Work out the finished part from the listing and answer in its coordinate system (mm). Round coordinates to 2 decimals unless told otherwise and drop trailing zeros. Write each loop counter-clockwise with the first axis right and the second up, starting at its lowest first coordinate (ties: lowest second). Pieces come first, ordered by that corner, then holes. Notation, with made-up numbers: (44, 26.5) -> (101, 26.5) arc R5 cw to (101, 33.5) -> close; hole circle Ø11 at (43.25, -35). An arc over 180 degrees is marked (long way). Answer as a JSON object with one key per item and string values. Group by question number.
from build123d import *

# Parameters (mm, degrees)
EXTRUDE_1_DEPTH      = 3
CUT_EXTRUDE_2_DEPTH  = 10
SKETCH_4_R           = 1.5
CUT_EXTRUDE_3_DEPTH  = 10
CUT_EXTRUDE_6_DEPTH  = 327.235911434
SKETCH_12_W          = 293.771267283
SKETCH_12_H          = 20
EXTRUDE_2_DEPTH      = 3
SKETCH_13_R          = 2
CUT_EXTRUDE_9_DEPTH  = 278.623703749
CUT_EXTRUDE_10_DEPTH = 10
MM_2_D               = 1.5
CUT_EXTRUDE_11_DEPTH = 278.623703749
MM_3_D               = 1.5
FILLET_1_R           = 2


with BuildPart() as part:
    # 草图1 → 凸台-拉伸1 (new body)
    with BuildSketch(Plane.XY):
        Polygon((-31.770103996, 71.767703031), (318.229896004, 71.767703031), (292.931935015, -47.249845949), (-31.770103996, 21.767703031), align=None)
    extrude(amount=EXTRUDE_1_DEPTH)

    # 草图3 → 切除-拉伸2 (cut)
    with BuildSketch(Plane.XY.offset(3)):
        Polygon((-0.469380772, 15.114528924), (0.1543543, 18.048971727), (-31.770103996, 24.834724815), (-31.770103996, 21.767703031), align=None)
        Polygon((176.220922432, -19.375132621), (205.565350454, -25.612483345), (204.941615382, -28.546926147), (175.59718736, -22.309575423), align=None)
    extrude(amount=-CUT_EXTRUDE_2_DEPTH, mode=Mode.SUBTRACT)

    # 草图4 → 切除-拉伸3 (cut)
    with BuildSketch(Plane.XY.offset(3)):
        with Locations((-20.141101902, 42.809716012)):
            Circle(SKETCH_4_R)
        with Locations((-0.578149887, 38.651482195)):
            Circle(SKETCH_4_R)
        with Locations((185.269894252, -0.85173906)):
            Circle(SKETCH_4_R)
        with Locations((204.832846267, -5.009972876)):
            Circle(SKETCH_4_R)
    extrude(amount=-CUT_EXTRUDE_3_DEPTH, mode=Mode.SUBTRACT)

    # 草图7 → 切除-拉伸6 (cut, through all)
    with BuildSketch(Plane.XY.offset(3)):
        Polygon((292.931935015, -47.249845949), (239.133816975, -35.814702954), (262.001163287, 71.767703031), (318.229896004, 71.767703031), align=None)
    extrude(amount=-CUT_EXTRUDE_6_DEPTH, mode=Mode.SUBTRACT)

    # 草图12 → 凸台-拉伸2 (add)
    with BuildSketch(Plane.XY.offset(3)):
        with Locations((115.115529646, 81.767703031)):
            Rectangle(SKETCH_12_W, SKETCH_12_H)
    extrude(amount=-EXTRUDE_2_DEPTH)

    # 草图13 → 切除-拉伸9 (cut, through all)
    with BuildSketch(Plane.XY.offset(3)):
        with Locations((-6.770103996, 81.767703031)):
            Circle(SKETCH_13_R)
        with Locations((73.229896004, 81.767703031)):
            Circle(SKETCH_13_R)
        with Locations((153.229896004, 81.767703031)):
            Circle(SKETCH_13_R)
        with Locations((233.229896004, 81.767703031)):
            Circle(SKETCH_13_R)
    extrude(amount=-CUT_EXTRUDE_9_DEPTH, mode=Mode.SUBTRACT)

    # 草图14 → 切除-拉伸10 (cut)
    with BuildSketch(Plane.XY.offset(3)):
        with BuildLine():
            Line((33.229896004, 67.767703031), (213.229896004, 67.767703031))
            ThreePointArc((213.229896004, 67.767703031), (221.229896004, 59.767703031), (213.229896004, 51.767703031))
            Line((213.229896004, 51.767703031), (33.229896004, 51.767703031))
            ThreePointArc((33.229896004, 51.767703031), (25.229896004, 59.767703031), (33.229896004, 67.767703031))
        make_face()
        with BuildLine():
            Line((53.229896004, 35.767703031), (223.229896004, 35.767703031))
            ThreePointArc((223.229896004, 35.767703031), (229.229896004, 29.767703031), (223.229896004, 23.767703031))
            Line((223.229896004, 23.767703031), (53.229896004, 23.767703031))
            ThreePointArc((53.229896004, 23.767703031), (47.229896004, 29.767703031), (53.229896004, 35.767703031))
        make_face()
    extrude(amount=-CUT_EXTRUDE_10_DEPTH, mode=Mode.SUBTRACT)

    # 大小mm 暗销槽口2 (through all)
    with Locations(Plane.XY.offset(3)):
        with Locations((0.1543543, 18.048971727), (176.220922432, -19.375132621), (205.565350454, -25.612483345)):
            Hole(MM_2_D / 2)

    # 草图18 → 切除-拉伸11 (cut, through all)
    with BuildSketch(Plane(origin=(0, 0, 0), x_dir=(-1, 0, 0), z_dir=(0, 0, -1))):
        Polygon((-152.291642964, -11.221785469), (-151.667907892, -14.156228271), (-122.32347987, -7.918877547), (-122.947214942, -4.984434744), align=None)
        Polygon((-64.258358898, 7.490266705), (-63.634623826, 4.555823902), (-34.290195804, 10.793174627), (-34.913930876, 13.727617429), align=None)
    extrude(amount=-CUT_EXTRUDE_11_DEPTH, mode=Mode.SUBTRACT)

    # 大小mm 暗销槽口3 (through all)
    with Locations(Plane(origin=(0, 0, 0), x_dir=(-1, 0, 0), z_dir=(0, 0, -1))):
        with Locations((-152.291642964, -11.221785469), (-151.667907892, -14.156228271), (-122.32347987, -7.918877547), (-122.947214942, -4.984434744), (-64.258358898, 7.490266705), (-63.634623826, 4.555823902), (-34.290195804, 10.793174627), (-34.913930876, 13.727617429)):
            Hole(MM_3_D / 2)

    # 圆角1
    fillet_1_edges = [part.edges().sort_by_distance(p)[0] for p in [
        (-31.770103996, 24.834724815, 1.5),
        (239.133816975, -35.814702954, 1.5),
        (262.001163287, 71.767703031, 1.5),
        (-31.770103996, 91.767703031, 1.5),
        (262.001163287, 91.767703031, 1.5),
    ]]
    fillet(fillet_1_edges, radius=FILLET_1_R)


solid = part.part
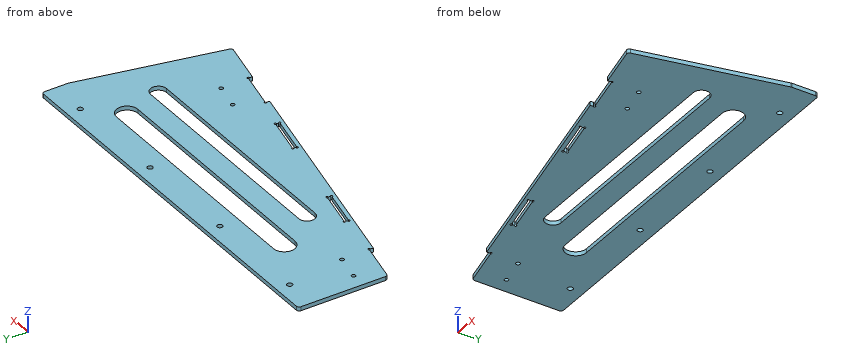
1) A cutting plane is placed at D-D on z = 2.1. State how many separate pieces and enclosed holes the cut face has, plus the area to 3 significant figures.
2) A cutting plane is placed at B-B on x = 168.5. Determine the outline of the cut face in (y, z), plus the area to 3 significant figures.
3) A cutting plane is placed at C-C on x = 137. Determine the outline of the cut face in (y, z), plus the area to 3 significant figures.
4) Straight lines are drawn through the part: L1, parallel to Y at x = 179.5, z = 0.5; L2, parallel to Y at x = 93, z = 0.9; L3, parallel to Y at x = 139, z = 1.1. For each, find the intervals that lie inside material, in ascending order.
5) A cutting plane is placed at A-A on y = 56. Determine the outline of the cut face in (x, z).
6) This flat-tipped pin is pushed along its axis until it touches: P1, Ø1, axis at y = 63.5, z = 0.5, coming from the +X side. Where does it stop, or does it pass through?
Established:
{
 "1": {"separate pieces": "1", "enclosed holes": "12", "area": "22,800 mm²"},
 "2": {"outline": "(-20.8, 0) -> (23.77, 0) -> (23.77, 3) -> (-20.8, 3) -> close; (35.77, 0) -> (51.77, 0) -> (51.77, 3) -> (35.77, 3) -> close; (67.77, 0) -> (91.77, 0) -> (91.77, 3) -> (67.77, 3) -> close", "area": "254 mm²"},
 "3": {"outline": "(-14.11, 0) -> (-11.04, 0) -> (-11.04, 3) -> (-14.11, 3) -> close; (-7.97, 0) -> (23.77, 0) -> (23.77, 3) -> (-7.97, 3) -> close; (35.77, 0) -> (51.77, 0) -> (51.77, 3) -> (35.77, 3) -> close; (67.77, 0) -> (91.77, 0) -> (91.77, 3) -> (67.77, 3) -> close", "area": "224 mm²"},
 "4": {"L1": "y = -20.07 to 23.77, 35.77 to 51.77, 67.77 to 91.77", "L2": "y = -4.75 to 23.77, 35.77 to 51.77, 67.77 to 91.77", "L3": "y = -14.53 to -11.46, -8.4 to 23.77, 35.77 to 51.77, 67.77 to 91.77"},
 "5": {"outline": "(-31.77, 0) -> (26.17, 0) -> (26.17, 3) -> (-31.77, 3) -> close; (220.29, 0) -> (258.65, 0) -> (258.65, 3) -> (220.29, 3) -> close"},
 "6": {"P1": "stops at x = 260.35"}
}
